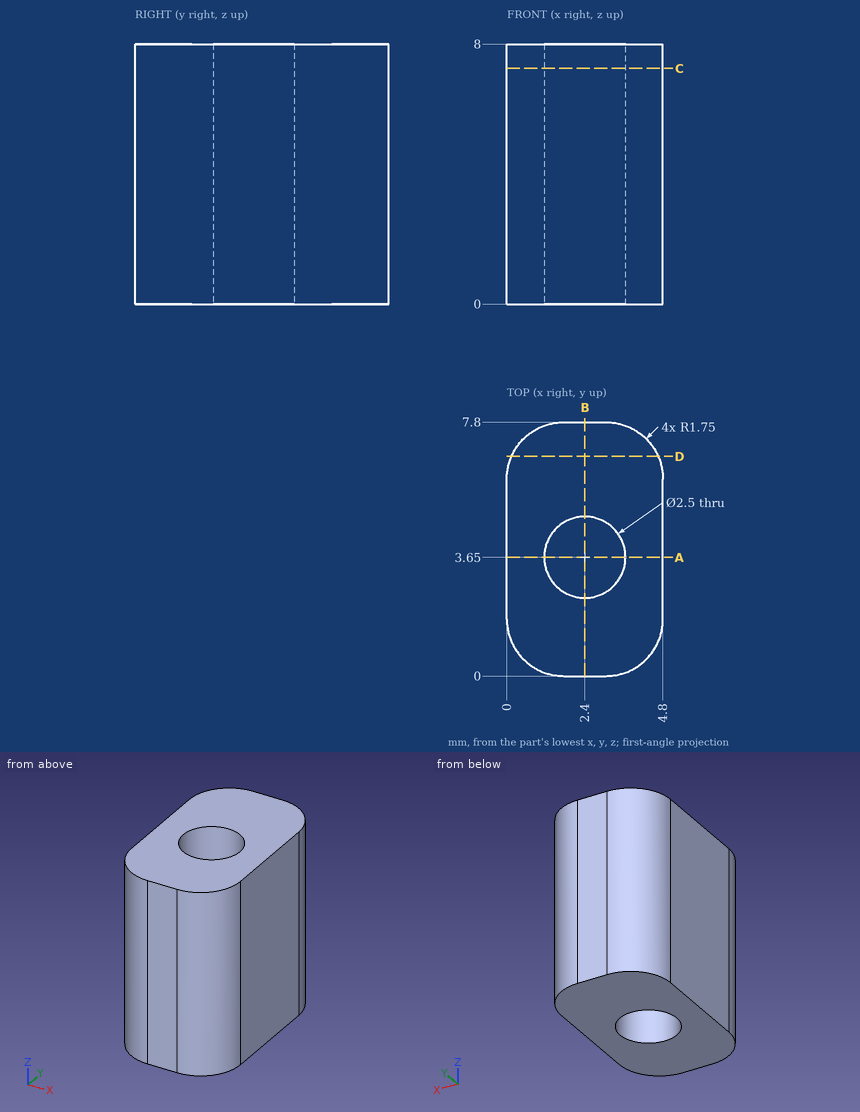
Study the drawing (mm; zero at the part's minimum x, y, z) and answer. Give positions to 0.01 mm unless a question says otherwise; leave off trailing zeros. Loops run counter-clockwise (first coordinate to the right, second up) from the corner with the lowest first, then second, coordinate; pieces in that order, holes last. Notation, with made-up numbers: (-17, -7) -> (12, -7) arc R28 ccw to (12, 24) -> close; hole circle Ø7 at (42, -2). An arc over 180 degrees is marked (long way). Use a Markdown table: item, result. Add a question column.
1) The part is cut by section B-B, the plane x = 2.4. Determine the outline of the cut face in (y, z).
2) Consider line 1 along Y through (x, z) = (2.4, 3.5); line 2 along Y through (x, z) = (1.8, 1.5); line 3 along X through (y, z) = (3.25, 1.25). Determine where each line is inside the solid, lowest interval first.
3) The part is cut by section C-C, the plane z = 7.25. Determine the outline of the cut face in (x, y), plus the area to 3 significant figures.
4) The part is cut by section A-A, the plane y = 3.65. Determine the outline of the cut face in (x, z).
5) Each of these flat-tipped pins is pushed along its axis until it touches: P1, Ø1.5, axis at x = 2.4, y = 3.65, coming from the -Z side; P2, Ø1.5, axis at x = 0.5, z = 5, coming from the -Y side. Where does it stop, or does it pass through?
6) The part is cut by section D-D, the plane y = 6.75. Determine the outline of the cut face in (x, z).
Reported:
| question | item | result |
|---|---|---|
| 1 | outline | (0, 0) -> (2.4, 0) -> (2.4, 8) -> (0, 8) -> close; (4.9, 0) -> (7.8, 0) -> (7.8, 8) -> (4.9, 8) -> close |
| 2 | line 1 | y = 0 to 2.4, 4.9 to 7.8 |
| 2 | line 2 | y = 0 to 2.55, 4.75 to 7.8 |
| 2 | line 3 | x = 0 to 1.22, 3.58 to 4.8 |
| 3 | outline | (0, 1.75) arc R1.75 ccw to (1.75, 0) -> (3.05, 0) arc R1.75 ccw to (4.8, 1.75) -> (4.8, 6.05) arc R1.75 ccw to (3.05, 7.8) -> (1.75, 7.8) arc R1.75 ccw to (0, 6.05) -> close; hole circle Ø2.5 at (2.4, 3.65) |
| 3 | area | 29.9 mm^2 |
| 4 | outline | (0, 0) -> (1.15, 0) -> (1.15, 8) -> (0, 8) -> close; (3.65, 0) -> (4.8, 0) -> (4.8, 8) -> (3.65, 8) -> close |
| 5 | P1 | passes through |
| 5 | P2 | stops at y = 0.07 |
| 6 | outline | (0.15, 0) -> (4.65, 0) -> (4.65, 8) -> (0.15, 8) -> close |
